Check sheet for the modelled part. Datum: model origin and axes. Units: mm. Give positions to 0.01 mm unless a question says otherwise; leave off trailing zeros. Return JSON: item names as keys, results as strings. Group by question number.
```python
from build123d import *

# Parameters (mm, degrees)
SKETCH1_R           = 14.2875
BOSS_EXTRUDE1_DEPTH = 12.7
FILLET1_R           = 0.79375


with BuildPart() as part:
    # Sketch1 → Boss-Extrude1 (new body, symmetric)
    with BuildSketch(Plane(origin=(0, 0, 0), x_dir=(0, 0, -1), z_dir=(1, 0, 0))):
        Circle(SKETCH1_R)
        Polygon((0.75, -1.299038106), (1.5, 0), (0.75, 1.299038106), (-0.75, 1.299038106), (-1.5, 0), (-0.75, -1.299038106), align=None, mode=Mode.SUBTRACT)
        with BuildLine():
            Line((3.175, 1.5875), (10.040231571, 1.5875))
            ThreePointArc((10.040231571, 1.5875), (10.6629003, 1.888987147), (10.812557076, 2.564423077))
            ThreePointArc((10.812557076, 2.564423077), (5.55625, 9.6237073), (-3.185423008, 10.646160647))
            ThreePointArc((-3.185423008, 10.646160647), (-3.695539293, 10.178836111), (-3.645300457, 9.4888456))
            Line((-3.645300457, 9.4888456), (-0.212684671, 3.543380657))
            ThreePointArc((-0.212684671, 3.543380657), (0.037374782, 3.277861812), (0.379778394, 3.152204526))
            ThreePointArc((0.379778394, 3.152204526), (1.5875, 2.749630657), (2.54, 1.905))
            ThreePointArc((2.54, 1.905), (2.820024209, 1.671298417), (3.175, 1.5875))
        make_face(mode=Mode.SUBTRACT)
        with BuildLine():
            Line((3.175, -1.5875), (10.040231571, -1.5875))
            ThreePointArc((10.040231571, -1.5875), (10.6629003, -1.888987147), (10.812557076, -2.564423077))
            ThreePointArc((10.812557076, -2.564423077), (5.55625, -9.6237073), (-3.185423008, -10.646160647))
            ThreePointArc((-3.185423008, -10.646160647), (-3.695539293, -10.178836111), (-3.645300457, -9.4888456))
            Line((-3.645300457, -9.4888456), (-0.212684671, -3.543380657))
            ThreePointArc((-0.212684671, -3.543380657), (0.037374782, -3.277861812), (0.379778394, -3.152204526))
            ThreePointArc((0.379778394, -3.152204526), (1.5875, -2.749630657), (2.54, -1.905))
            ThreePointArc((2.54, -1.905), (2.820024209, -1.671298417), (3.175, -1.5875))
        make_face(mode=Mode.SUBTRACT)
        with BuildLine():
            Line((-2.962315329, -1.955880657), (-6.394931114, -7.9013456))
            ThreePointArc((-6.394931114, -7.9013456), (-6.967361007, -8.289848964), (-7.627134069, -8.08173757))
            ThreePointArc((-7.627134069, -8.08173757), (-11.1125, 0), (-7.627134069, 8.08173757))
            ThreePointArc((-7.627134069, 8.08173757), (-6.967361007, 8.289848964), (-6.394931114, 7.9013456))
            Line((-6.394931114, 7.9013456), (-2.962315329, 1.955880657))
            ThreePointArc((-2.962315329, 1.955880657), (-2.857398991, 1.606563395), (-2.919778394, 1.247204526))
            ThreePointArc((-2.919778394, 1.247204526), (-3.175, 0), (-2.919778394, -1.247204526))
            ThreePointArc((-2.919778394, -1.247204526), (-2.857398991, -1.606563395), (-2.962315329, -1.955880657))
        make_face(mode=Mode.SUBTRACT)
    extrude(amount=BOSS_EXTRUDE1_DEPTH, both=True)

    # Fillet1
    fillet1_edges = [part.edges().sort_by_distance(p)[0] for p in [
        (-12.7, 0, 14.2875),
        (12.7, 0, 14.2875),
    ]]
    fillet(fillet1_edges, radius=FILLET1_R)


solid = part.part
```
Item 1: Material ranges on line 1 along Z through (x, y) = (7.25, 8); line 2 along Y through (x, z) = (-1, -6.5); line 3 along Z through (x, y) = (1.75, -5.5), recorded low to high. Write a range as from..to.
Item 2: Mould release check, pull along Z, two halves, no side actions. Record for faces 1 (the face through (12.7, -3, 0)), 2 (the face through (0.167, 0.628, 14.274)), 3 (the face through (0.178, 1.881, -10.657)), 4 (the face through (0.178, -1.881, -10.657)): +Z half, -Z half, draft (parallel to the pull), parting line (faces both ways), or undercut.
Item 3: Depth check by flat-ended pin: pin 1 (8 mm diameter, centred on x = -10, z = -2, fed in from +Y); pin 2 (2 mm diameter, centred on x = 2, z = -8, fed in from +Y); pin 3 (4 mm diameter, centred on y = 8, z = -0.5, fed in from -X); pin 4 (1 mm diameter, centred on x = -1, z = 6, fed in from -Y). Enter the tip coordinate at first touch or a pass-through.
Item 4: Section check A-A on x = 8. Count the separate pieces of the cut face and the enclosed holes in it, plus the area to 3 significant figures.
Reply:
{
 "1": {"line 1": "-11.84..-7.71, 2.79..6.46, 7.71..11.84", "line 2": "-12.72..-9.01, -1.59..1.59, 9.01..12.72", "line 3": "-13.19..-9.66, 1.34..5.01, 9.66..13.19"},
 "2": {"face 1": "draft", "face 2": "parting line", "face 3": "undercut", "face 4": "undercut"},
 "3": {"pin 1": "y = 14.29", "pin 2": "y = 12.46", "pin 3": "through", "pin 4": "y = -13.19"},
 "4": {"separate pieces": "1", "enclosed holes": "4", "area": "357 mm²"}
}
